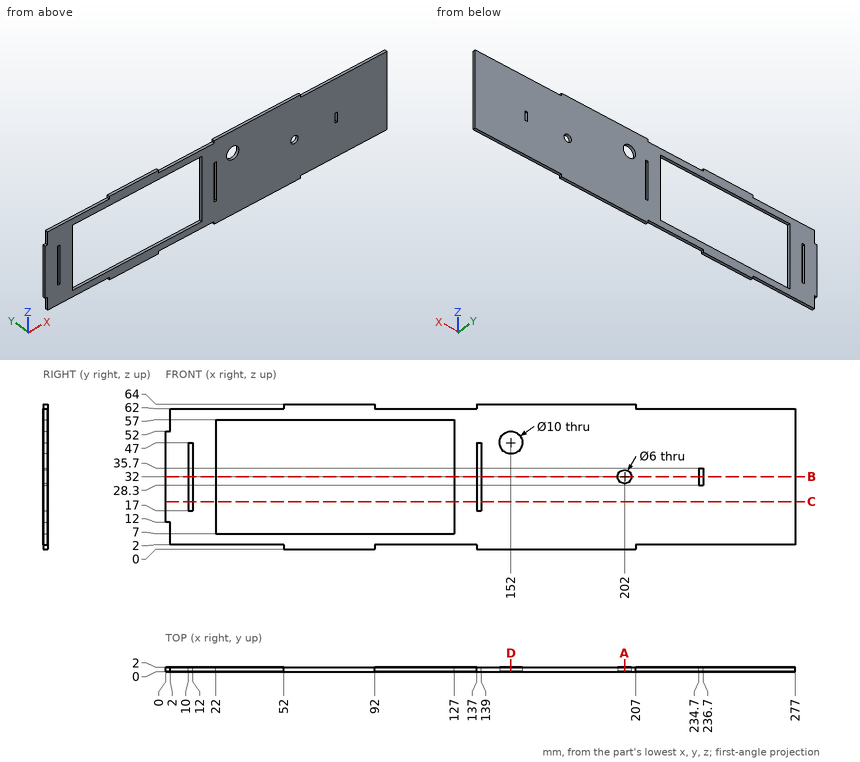
Study the drawing (mm; zero at the part's minimum x, y, z) and answer. Give positions to 0.01 mm unless a question says otherwise; leave off trailing zeros. Write each loop counter-clockwise with the first axis right and the second up, starting at its lowest first coordinate (ties: lowest second). Pieces come first, ordered by that corner, then holes. Notation, with made-up numbers: (-36, -26.75) -> (-7, -26.75) arc R6 ccw to (-7, -20.75) -> close; hole circle Ø9 at (-0.5, 67). An arc over 180 degrees is marked (long way). Write item = value, one per line.
Q1. Section D-D on x = 152 is taken. Determine the outline of the cut face in (y, z).
Computed values:
outline = (0, 0) -> (2, 0) -> (2, 42) -> (0, 42) -> close; (0, 52) -> (2, 52) -> (2, 64) -> (0, 64) -> close
Q2. Section B-B on z = 32 is taken. Determine the outline of the cut face in (x, y).
Computed values:
outline = (0, 0) -> (10, 0) -> (10, 2) -> (0, 2) -> close; (12, 0) -> (22, 0) -> (22, 2) -> (12, 2) -> close; (127, 0) -> (137, 0) -> (137, 2) -> (127, 2) -> close; (139, 0) -> (199, 0) -> (199, 2) -> (139, 2) -> close; (205, 0) -> (234.7, 0) -> (234.7, 2) -> (205, 2) -> close; (236.7, 0) -> (277, 0) -> (277, 2) -> (236.7, 2) -> close
Q3. Section A-A on x = 202 is taken. Determine the outline of the cut face in (y, z).
Computed values:
outline = (0, 0) -> (2, 0) -> (2, 29) -> (0, 29) -> close; (0, 35) -> (2, 35) -> (2, 64) -> (0, 64) -> close
Q4. Section C-C on z = 21 is taken. Determine the outline of the cut face in (x, y), and give its area (3 significant figures).
Computed values:
outline = (0, 0) -> (10, 0) -> (10, 2) -> (0, 2) -> close; (12, 0) -> (22, 0) -> (22, 2) -> (12, 2) -> close; (127, 0) -> (137, 0) -> (137, 2) -> (127, 2) -> close; (139, 0) -> (277, 0) -> (277, 2) -> (139, 2) -> close
area = 336 mm^2
Q5. Consider line 1 along X through (y, z) = (1.6, 32); line 2 along X through (y, z) = (1.4, 28); line 3 along Z through (x, y) = (152, 0.85). Determine where each line is inside the solid, lowest interval first.
Computed values:
line_1 = 0 to 10, 12 to 22, 127 to 137, 139 to 199, 205 to 234.7, 236.7 to 277
line_2 = 0 to 10, 12 to 22, 127 to 137, 139 to 277
line_3 = 0 to 42, 52 to 64
Q6. Flat-ended cylindrical pins translate along their axes: pin 1 Ø1 at (x, y) = (11, 1) entering from -Z; pin 2 Ø0.6 at (y, z) = (1, 63) entering from +X; pin 3 Ø0.6 at (y, z) = (1, 58.5) entering from -X. Find the tip coordinate at first contact, or state that the pin passes through.
Computed values:
pin_1 = 2
pin_2 = 207
pin_3 = 2
